Read the model definition and answer for the solid it produces. Units are mm, in the model's axes. Face numbers are marked on the shaded views. A direction names the side the tool comes from. Give positions to 0.01 mm unless a question says otherwise; leave off trailing zeros. Order: outer loops, then holes, each group sorted by start corner. A loop starts at its lowest first (then second) coordinate and runs counter-clockwise, first axis right, second up. Notation, with made-up numbers: (13, 39) - (58, 39) arc R22 ccw to (58, 61) - close; hole circle Ø11 at (-8.75, -39). An arc over 180 degrees is marked (long way). Write item = value, one per line.
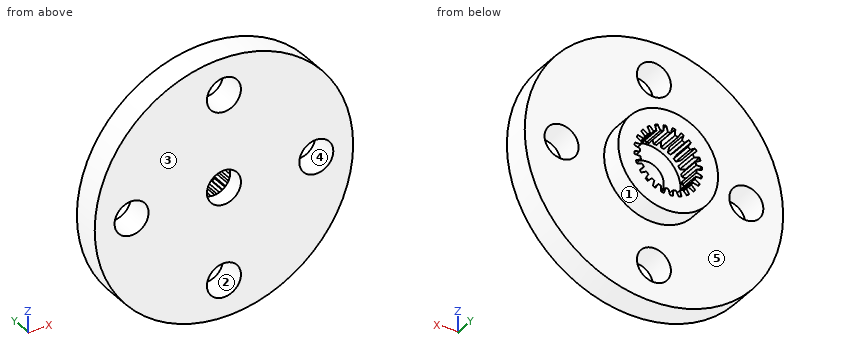
```python
from build123d import *

# Parameters (mm, degrees)
SKETCH_4_R               = 11.4
EXTRUDE_2_DEPTH          = 2.5
SKETCH_6_R               = 1.5
CUT_EXTRUDE_9_DEPTH      = 2.5
SKETCH_7_R               = 4.4
EXTRUDE_3_DEPTH          = 2
SKETCH_8_R               = 3
CUT_EXTRUDE_10_DEPTH     = 3
EXTRUDE_5_DEPTH          = 2
PATTERN_CIRCULAR_1_COUNT = 24


with BuildPart() as part:
    # Sketch 4 → Extrude 2 (new body)
    with BuildSketch(Plane(origin=(0, 0, 0), x_dir=(1, 0, 0), z_dir=(0, 1, 0))):
        Circle(SKETCH_4_R)
    extrude(amount=EXTRUDE_2_DEPTH)

    # Sketch 6 → Cut-Extrude 9 (cut)
    with BuildSketch(Plane(origin=(0, 2.5, 0), x_dir=(1, 0, 0), z_dir=(0, 1, 0))):
        with Locations((0, 8.15)):
            Circle(SKETCH_6_R)
        Circle(SKETCH_6_R)
        with Locations((8.15, 0)):
            Circle(SKETCH_6_R)
        with Locations((-8.15, 0)):
            Circle(SKETCH_6_R)
        with Locations((0, -8.15)):
            Circle(SKETCH_6_R)
    extrude(amount=-CUT_EXTRUDE_9_DEPTH, mode=Mode.SUBTRACT)

    # Sketch 7 → Extrude 3 (add)
    with BuildSketch(Plane(origin=(0, 2.5, 0), x_dir=(1, 0, 0), z_dir=(0, 1, 0))):
        Circle(SKETCH_7_R)
    extrude(amount=EXTRUDE_3_DEPTH)

    # Sketch 8 → Cut-Extrude 10 (cut)
    with BuildSketch(Plane(origin=(0, 4.5, 0), x_dir=(1, 0, 0), z_dir=(0, 1, 0))):
        Circle(SKETCH_8_R)
    extrude(amount=-CUT_EXTRUDE_10_DEPTH, mode=Mode.SUBTRACT)

    # Sketch 14 → Extrude 5 (add)
    with BuildSketch(Plane(origin=(0, 4.5, 0), x_dir=(1, 0, 0), z_dir=(0, 1, 0))):
        with BuildLine():
            Line((2.976910005, -0.371492698), (2.495792863, -0.23538136))
            Line((2.495792863, -0.23538136), (2.495792863, 0.032272898))
            Line((2.495792863, 0.032272898), (2.995792863, 0.158824181))
            ThreePointArc((2.995792863, 0.158824181), (2.998100046, -0.106752588), (2.976910005, -0.371492698))
        make_face()
    extrude_5 = extrude(amount=-EXTRUDE_5_DEPTH)

    # Pattern Circular 1: Extrude 5 ×24 about axis
    pattern_circular_1_axis = Axis((0, 0, 0), (0, 1, 0))
    for i in range(1, PATTERN_CIRCULAR_1_COUNT):
        add(extrude_5.rotate(pattern_circular_1_axis, i * 360 / PATTERN_CIRCULAR_1_COUNT))


solid = part.part
```
1. For the marked faces 4 and 5, determine the directions among +Z, -Z, +X, -X, +Y, -Y from which every point of the face is accessible in a straight line to the end or side of a thin tool.
Recorded:
face_4 = +Y, -Y
face_5 = +Y
2. Straight lines are drawn through the part: L1, parallel to Z at x = 0, y = 1.9; L2, parallel to Z at x = 0, y = 0.75. For each, find the intervals that lie inside material, in ascending order. Write a range as [from, to].
Recorded:
L1 = [-11.4, -9.65], [-6.65, -3], [3, 6.65], [9.65, 11.4]
L2 = [-11.4, -9.65], [-6.65, -1.5], [1.5, 6.65], [9.65, 11.4]
3. Flat-ended cylindrical pins translate along their axes: pin 1 (5 mm diameter, centred on x = 0, z = 0, fed in from -Y); pin 2 (3.5 mm diameter, centred on x = 0, z = 0, fed in from +Y). Find the tip coordinate at first contact, or state that the pin passes through.
Recorded:
pin_1 = 0
pin_2 = 1.5
4. Determine the mould class of the marked faces 1, 2 and 3 for opening direction Z: +Z half, -Z half, draft (parallel to the pull), parting line (faces both ways), or undercut.
Recorded:
face_1 = parting line
face_2 = undercut
face_3 = draft
5. Section B-B (z = 7.25) is taken. Determine the outline of the cut face in (x, y), and give its area (3 significant figures).
Recorded:
outline = (-8.8, 0) - (-1.2, 0) - (-1.2, 2.5) - (-8.8, 2.5) - close; (1.2, 0) - (8.8, 0) - (8.8, 2.5) - (1.2, 2.5) - close
area = 38.0 mm^2
6. Section C-C (z = -4.75) is taken. Determine the outline of the cut face in (x, y), and give its area (3 significant figures).
Recorded:
outline = (-10.36, 0) - (10.36, 0) - (10.36, 2.5) - (-10.36, 2.5) - close
area = 51.8 mm^2
7. Section A-A (x = 8.75) is taken. Determine the outline of the cut face in (y, z), and give its area (3 significant figures).
Recorded:
outline = (0, -7.31) - (2.5, -7.31) - (2.5, -1.37) - (0, -1.37) - close; (0, 1.37) - (2.5, 1.37) - (2.5, 7.31) - (0, 7.31) - close
area = 29.7 mm^2
